from build123d import *

# Parameters (mm, degrees)
F1_DEPTH  = 9
F3_DEPTH  = 6
F4_R      = 4
F5_DEPTH  = 25
F6_R      = 1.99999
F7_W      = 12
F7_H      = 6
F8_DEPTH  = 15
F9_W      = 12
F9_H      = 5
F10_DEPTH = 25


# Not quite as in the source:
# - a fillet or chamfer is up to 0.001 mm smaller than in the source, because OpenCascade refuses the exact size


with BuildPart() as f1:
    # F0 (on Front) → F1 (new body)
    with BuildSketch(Plane.XZ):
        with BuildLine():
            ThreePointArc((0, 44), (-15.9099025767, 37.4099025767), (-22.5, 21.5))
            Line((-22.5, 21.5), (0, 21.5))
            Line((0, 21.5), (0, 44))
        make_face()
        with BuildLine():
            ThreePointArc((0, -1), (-15.9099025767, 5.5900974233), (-22.5, 21.5))
            Line((-22.5, 21.5), (-22.5, -21.5))
            Line((-22.5, -21.5), (0, -21.5))
            Line((0, -21.5), (0, -1))
        make_face()
        with BuildLine():
            Line((0, 21.5), (-22.5, 21.5))
            ThreePointArc((-22.5, 21.5), (-15.9099025767, 5.5900974233), (0, -1))
            Line((0, -1), (0, 21.5))
        make_face()
        with BuildLine():
            Line((0, 44), (0, 21.5))
            Line((0, 21.5), (22.5, 21.5))
            ThreePointArc((22.5, 21.5), (15.9099025767, 37.4099025767), (0, 44))
        make_face()
        with BuildLine():
            Line((22.5, 21.5), (0, 21.5))
            Line((0, 21.5), (0, -1))
            ThreePointArc((0, -1), (15.9099025767, 5.5900974233), (22.5, 21.5))
        make_face()
        with BuildLine():
            ThreePointArc((22.5, 21.5), (15.9099025767, 5.5900974233), (0, -1))
            Line((0, -1), (0, -21.5))
            Line((0, -21.5), (22.5, -21.5))
            Line((22.5, -21.5), (22.5, 21.5))
        make_face()
    extrude(amount=F1_DEPTH)

    # F2 (on face) → F3 (cut)
    with BuildSketch(Plane.XZ.offset(9)):
        with BuildLine():
            Line((0, 30.8210086077), (0, 44))
            ThreePointArc((0, 44), (-2.5157755473, 43.8589103803), (-5, 43.4374109685))
            Line((-5, 43.4374109685), (-5, 30.8210086077))
            Line((-5, 30.8210086077), (0, 30.8210086077))
        make_face()
        with BuildLine():
            Line((0, 22), (0, 30.8210086077))
            Line((0, 30.8210086077), (-5, 30.8210086077))
            Line((-5, 30.8210086077), (-5, 20.7979589711))
            ThreePointArc((-5, 20.7979589711), (-2.5712303784, 21.695268783), (0, 22))
        make_face()
        with BuildLine():
            ThreePointArc((11, 11), (7.7781745931, 18.7781745931), (0, 22))
            ThreePointArc((0, 22), (-2.5712303784, 21.695268783), (-5, 20.7979589711))
            ThreePointArc((-5, 20.7979589711), (-8.3760412767, 3.8696470964), (8.8741196746, 4.5))
            ThreePointArc((8.8741196746, 4.5), (10.4550302826, 7.5805933571), (11, 11))
        make_face()
        with BuildLine():
            ThreePointArc((22.5, 21.5), (15.9099025767, 37.4099025767), (0, 44))
            Line((0, 44), (0, 30.8210086077))
            Line((0, 30.8210086077), (0, 22))
            ThreePointArc((0, 22), (7.7781745931, 18.7781745931), (11, 11))
            ThreePointArc((11, 11), (10.4550302826, 7.5805933571), (8.8741196746, 4.5))
            Line((8.8741196746, 4.5), (22.5, 4.5))
            Line((22.5, 4.5), (22.5, 21.5))
        make_face()
    extrude(amount=-F3_DEPTH, mode=Mode.SUBTRACT)

    # F4 (on face) → F5 (cut)
    with BuildSketch(Plane.XZ.offset(3)):
        with BuildLine():
            ThreePointArc((-4, 21.246950766), (6.204836823, 20.0829510623), (11, 11))
            ThreePointArc((11, 11), (10.7566660599, 8.6991012027), (10.0374299499, 6.5))
            Line((10.0374299499, 6.5), (14.3090880213, 6.5))
            ThreePointArc((14.3090880213, 6.5), (14.8262658872, 8.7236345108), (15, 11))
            ThreePointArc((15, 11), (9.0829510623, 22.9373363863), (-4, 25.4568322948))
            Line((-4, 25.4568322948), (-4, 21.246950766))
        make_face()
        with Locations((0, 11)):
            Circle(F4_R)
    extrude(amount=-F5_DEPTH, mode=Mode.SUBTRACT)

    # F6 (radius 2 in the source; OpenCascade refuses exactly that, so slightly less here)
    f6_edges = [f1.edges().sort_by_distance(p)[0] for p in [
        (-4, -1.5, 25.456832),
        (-4, -1.5, 21.246951),
        (14.309088, -1.5, 6.5),
        (10.03743, -1.5, 6.5),
    ]]
    fillet(f6_edges, radius=F6_R)

    # F7 (on face) → F8 (cut)
    with BuildSketch(Plane.XY.offset(4.5)):
        with Locations((14.5, -6)):
            Rectangle(F7_W, F7_H)
    extrude(amount=-F8_DEPTH, mode=Mode.SUBTRACT)

    # F9 (on face) → F10 (cut)
    with BuildSketch(Plane.XZ.offset(3)):
        with Locations((14.5, -8)):
            Rectangle(F9_W, F9_H)
    extrude(amount=-F10_DEPTH, mode=Mode.SUBTRACT)


solid = f1.part
Here's how the part is built. I have some questions about the finished solid (model axes, mm). A direction names the side the tool comes from. Give positions to 0.01 mm unless a question says otherwise; leave off trailing zeros. Loops run counter-clockwise (first coordinate to the right, second up) from the corner with the lowest first, then second, coordinate; pieces in that order, holes last. Notation, with made-up numbers: (-8, -9) -> (46, -9) arc R23 ccw to (46, 30) -> close; hole circle Ø10 at (46.25, 21). An arc over 180 degrees is marked (long way). One line per item, written item: value.
Q1. Suppose I cut it at B-B on x = 0. Please give me the cut outline in (y, z).
Answers follow:
outline: (-9, -21.5) -> (0, -21.5) -> (0, 7) -> (-3, 7) -> (-3, 0) -> (-9, 0) -> close; (-3, 15) -> (0, 15) -> (0, 22) -> (-3, 22) -> close; (-3, 26) -> (0, 26) -> (0, 44) -> (-3, 44) -> close
Q2. If I drill on line 1 along Z through (x, y) = (0, -1.55); line 2 along X through (y, z) = (-1.25, 14.5); line 3 along Y through (x, z) = (19.5, 17), over which ranges is the centre line in solid material (lowest first)?
Answers follow:
line 1: -21.5 to 7, 15 to 22, 26 to 44
line 2: -22.5 to -1.94, 1.94 to 10.43, 14.59 to 22.5
line 3: -3 to 0
Q3. Suppose I cut it at D-D on y = -7. Please give me the cut outline in (x, z).
Answers follow:
outline: (-22.5, -21.5) -> (22.5, -21.5) -> (22.5, 4.5) -> (20.5, 4.5) -> (20.5, -10.5) -> (8.5, -10.5) -> (8.5, 4.02) arc R11 cw (long way) to (-5, 20.8) -> (-5, 43.44) arc R22.5 ccw to (-22.5, 21.5) -> close
Q4. Suppose I cut it at A-A on z = 13. Please give me the cut outline in (x, y), then the cut area to 3 significant figures.
Answers follow:
outline: (-22.5, -9) -> (-10.82, -9) -> (-10.82, -3) -> (-3.46, -3) -> (-3.46, 0) -> (-22.5, 0) -> close; (3.46, -3) -> (10.82, -3) -> (10.82, 0) -> (3.46, 0) -> close; (14.87, -3) -> (22.5, -3) -> (22.5, 0) -> (14.87, 0) -> close
area: 172 mm^2
Q5. We'd pull the mould along X, two halves only. Please class faces 1 (the face through (-7.229, -3.437, 42.807)), 2 (the face through (11.198, -1.479, 7.248)), 3 (the face through (21, -6, 4.5)): pulls with the +X half, pulls with the -X half, needs draft (parallel to the pull), parting line crosses it, or undercut.
Answers follow:
face 1: parting line crosses it
face 2: undercut
face 3: needs draft
Q6. I'm going to push flat-ended pins straight in: pin 1 Ø1 at (y, z) = (-3, 28.5) entering from +X; pin 2 Ø1.8 at (y, z) = (-7, 37.5) entering from +X; pin 3 Ø1 at (y, z) = (-6, 7.5) entering from +X. Where does each tip first touch, or does it pass through?
Answers follow:
pin 1: x = 21.54
pin 2: x = -5
pin 3: x = -10.25
Q7. On a 3-axis mill with a long thin cutter (end or side, diameter ignored), from which of +Z, -Z, +X, -X, +Y, -Y can I reach the whole of each face in a straight line? I mean faces 4 (the face through (22.5, -4, -5)), 5 (the face through (20.5, -6, -3)), 6 (the face through (-3.506, -1.479, 25.161)). Say none if no direction works.
Answers follow:
face 4: +Z, -Z, +X, +Y, -Y
face 5: -Y
face 6: +Y, -Y
Q8. Suppose I cut it at C-C on y = -1. State how many separate pieces and enclosed holes the cut face has, then the cut area to 3 significant figures.
Answers follow:
separate pieces: 1
enclosed holes: 3
area: 2,510 mm^2
